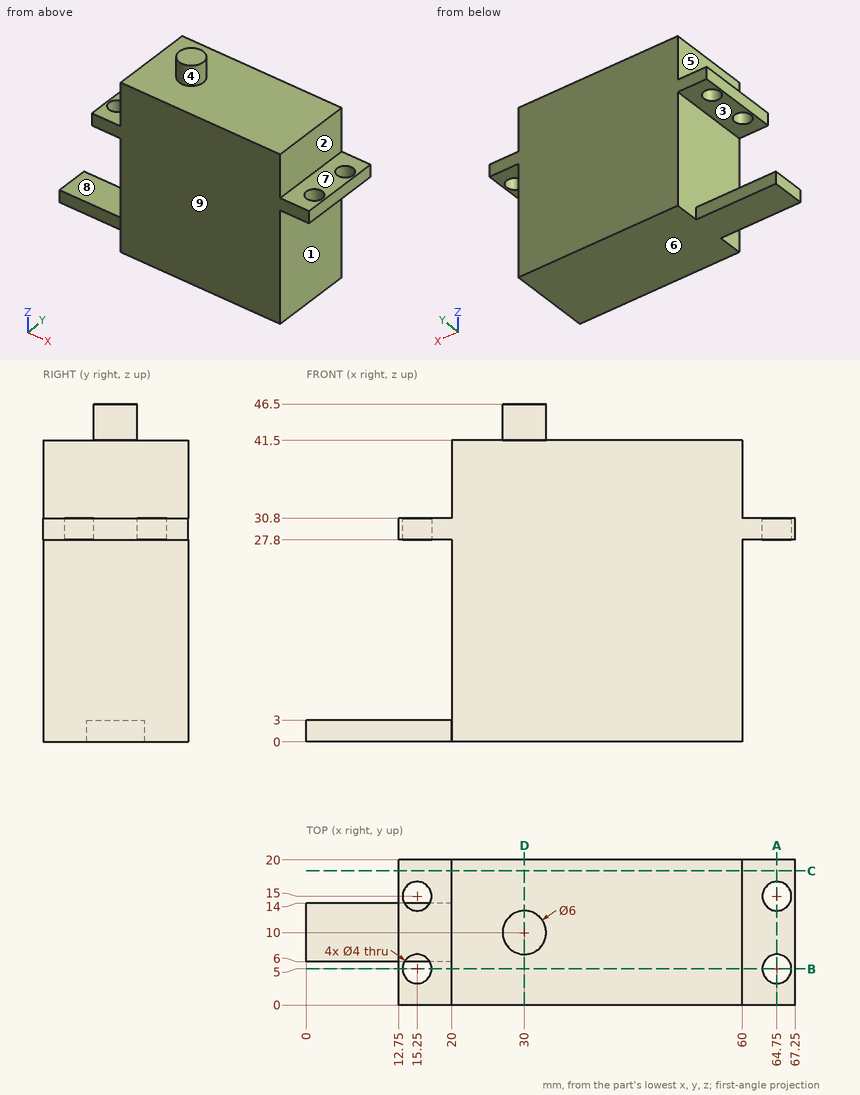
Here's the drawing with two shaded views (mm, measured from the low corner). I have some questions. A direction names the side the tool comes from. Coordinates: 2 decimals unless noted, no trailing zeros. Loops run counter-clockwise (first coordinate to the right, second up) from the corner with the lowest first, then second, coordinate; pieces in that order, holes last. Notation, with made-up numbers: (88.25, -6) -> (141.25, -6) arc R14 cw to (141.25, 16) -> close; hole circle Ø3 at (56, 32.5). An arc over 180 degrees is marked (long way). Put each result on its own line as item: value. Start each with the question number.
Q1. For the marked faces 1, 2, 3, 4 and 5, which set-ups out of +Z, -Z, +X, -X, +Y, -Y let a thin tool reach every point of the face, with its end or its side?
Q2. If I drill on line 1 (Y direction, x = 64.75, z = 29.75); line 2 (Y direction, x = 64, z = 29); line 3 (X direction, y = 5, z = 37.5), over which ranges is the centre line in solid material (lowest first)? Write a range as [from, to].
Q3. I want a section at D-D (x = 30). Write out the boundary of the cut face in (y, z), plus the area to 3 significant figures.
Q4. I'm going to push flat-ended pins straight in: P1, Ø1.5, axis at x = 40.5, y = 8, coming from the +Z side; P2, Ø12, axis at y = 14.5, z = 35.5, coming from the -X side; P3, Ø6, axis at y = 12.5, z = 18.5, coming from the -X side. Where does each tip first touch, or does it pass through?
Q5. I want a section at B-B (y = 5). Write out the boundary of the cut face in (x, z), plus the area to 3 significant figures.
Q6. Thinking about a two-plate mould opening in Z: for the marked faces 6, 7, 8 and 9, which applies, pulls with the +Z half, pulls with the -Z half, needs draft (parallel to the pull), parting line crosses it, or undercut?
Q7. I want a section at C-C (y = 18.5). Write out the boundary of the cut face in (x, z), plus the area to 3 significant figures.
Q8. I want a section at A-A (x = 64.75). Write out the boundary of the cut face in (y, z), plus the area to 3 significant figures.
Taken from the geometry:
1. face 1: -Z, +X, +Y, -Y
1. face 2: +Z, +X, +Y, -Y
1. face 3: -X, +Y, -Y
1. face 4: +Z
1. face 5: +Z, -X, +Y, -Y
2. line 1: y = [0, 3], [7, 13], [17, 20]
2. line 2: y = [0, 3.15], [6.85, 13.15], [16.85, 20]
2. line 3: x = [20, 60]
3. outline: (0, 0) -> (20, 0) -> (20, 41.5) -> (13, 41.5) -> (13, 46.5) -> (7, 46.5) -> (7, 41.5) -> (0, 41.5) -> close
3. area: 860 mm2
4. P1: stops at z = 41.5
4. P2: stops at x = 12.75
4. P3: stops at x = 20
5. outline: (12.75, 27.8) -> (13.25, 27.8) -> (13.25, 30.8) -> (12.75, 30.8) -> close; (17.25, 27.8) -> (20, 27.8) -> (20, 0) -> (60, 0) -> (60, 27.8) -> (62.75, 27.8) -> (62.75, 30.8) -> (60, 30.8) -> (60, 41.5) -> (20, 41.5) -> (20, 30.8) -> (17.25, 30.8) -> close; (66.75, 27.8) -> (67.25, 27.8) -> (67.25, 30.8) -> (66.75, 30.8) -> close
5. area: 1,680 mm2
6. face 6: pulls with the -Z half
6. face 7: pulls with the +Z half
6. face 8: undercut
6. face 9: needs draft
7. outline: (12.75, 27.8) -> (20, 27.8) -> (20, 0) -> (60, 0) -> (60, 27.8) -> (67.25, 27.8) -> (67.25, 30.8) -> (60, 30.8) -> (60, 41.5) -> (20, 41.5) -> (20, 30.8) -> (12.75, 30.8) -> close
7. area: 1,700 mm2
8. outline: (0, 27.8) -> (3, 27.8) -> (3, 30.8) -> (0, 30.8) -> close; (7, 27.8) -> (13, 27.8) -> (13, 30.8) -> (7, 30.8) -> close; (17, 27.8) -> (20, 27.8) -> (20, 30.8) -> (17, 30.8) -> close
8. area: 36.0 mm2
